Input: part model. Units: mm. Frame: model coordinates. A direction names the side the tool comes from. Round coordinates to 2 decimals unless told otherwise and drop trailing zeros. Loops run counter-clockwise (first coordinate to the right, second up) from the corner with the lowest first, then second, coordinate; pieces in that order, holes last. Notation, with made-up numbers: (-18, 30) -> (26, 30) arc R17 cw to (26, 63) -> close; hole circle Ø10 at (30, 15). An arc over 180 degrees is marked (long way). One line per question, with ' | ' between items. Start each with the question number.
Q1. Cut plane B-B on z = -33.5. Return loops of the section in (x, y).
Q2. Cut plane A-A on y = -32. Return loops of the section in (x, z), and give its area (3 significant figures).
Q3. Cut plane C-C on y = -54. Return loops of the section in (x, z).
Q4. Material intervals for L1, parallel to X at y = 14.5, z = -30.5; L2, parallel to X at y = -9, z = -60; L3, parallel to Y at x = 29, z = -35, sorted ascending.
Q5. Contact query for flat-ended pins moving along their axis: P1, Ø2, axis at y = -6, z = -55, coming from the -X side; P2, Ø10, axis at y = -37.5, z = -27.5, coming from the -X side; P3, Ø2, axis at x = 23, z = -21, coming from the +Y side. Output: stop coordinate, or through.
Q6. Access query for faces 4 (the face through (-49.361, -66.737, -34.51)), 5 (the face through (-32.41, -16.09, -34.51)). Directions: +Z, -Z, +X, -X, +Y, -Y. A direction counts if a zero-diameter tool reaches every point of the face in a straight line with its end or side. Return the directions, or none.
Q7. Mould query, pull axis Y, two halves, no side actions, for faces 1 (the face through (14, -4, -70)), 2 (the face through (-14.52, 54.31, -34.51)), 3 (the face through (19.58, -14.68, -34.51)). Classes: pulls with the +Y half, pulls with the -Y half, needs draft (parallel to the pull), parting line crosses it, or undercut.
Q8. Cut plane D-D on x = -28.5. Return loops of the section in (y, z).
from build123d import *

# Parameters (mm, degrees)
F1_DEPTH = 70


with BuildPart() as f1:
    # F0 (on Top) → F1 (new body)
    with BuildSketch(Plane.XY):
        Polygon((-53.090672, -65.789246), (-45.524913, -67.711686), (-18.916096, 37.007269), (59.177905, -67.84258), (64.177905, -67.84258), (-17.897495, 41.015974), (-11.04691, 67.976439), (-12.597631, 68.370474), (-46.085725, -63.421866), (-49.307792, -62.603147), (-48.913758, -61.052425), (-51.708323, -60.349014), (-52.100763, -61.89346), align=None)
    extrude(amount=-F1_DEPTH)


solid = f1.part
Results:
1) outline: (-53.09, -65.79) -> (-45.52, -67.71) -> (-18.92, 37.01) -> (59.18, -67.84) -> (64.18, -67.84) -> (-17.9, 41.02) -> (-11.05, 67.98) -> (-12.6, 68.37) -> (-46.09, -63.42) -> (-49.31, -62.6) -> (-48.91, -61.05) -> (-51.71, -60.35) -> (-52.1, -61.89) -> close
2) outline: (-38.1, -70) -> (-36.45, -70) -> (-36.45, 0) -> (-38.1, 0) -> close; (32.48, -70) -> (37.15, -70) -> (37.15, 0) -> (32.48, 0) -> close | area: 443 mm^2
3) outline: (-43.69, -70) -> (-42.04, -70) -> (-42.04, 0) -> (-43.69, 0) -> close; (48.87, -70) -> (53.74, -70) -> (53.74, 0) -> (48.87, 0) -> close
4) L1: -26.29 to -24.64, -2.15 to 2.09 | L2: -32.26 to -30.61, 15.35 to 19.81 | L3: -27.33 to -21.19
5) P1: x = -31.75 | P2: x = -40.77 | P3: y = -11.9
6) face 4: +Z, -Z, -X, -Y | face 5: +Z, -Z, -Y
7) face 1: needs draft | face 2: undercut | face 3: pulls with the -Y half
8) outline: (-0.71, -70) -> (5.79, -70) -> (5.79, 0) -> (-0.71, 0) -> close
